The listing builds one solid part. Answer for the finished solid, in the listing's coordinates (mm). Coordinates: 2 decimals unless noted, no trailing zeros. Answer as a JSON object with one key per item and string values. Group by question number.
from build123d import *

# Parameters (mm, degrees)
BOSS_EXTRUDE1_DEPTH         = 3.175
F_1_4_0_25_DIAMETER_HOLE1_D = 6.35
FILLET1_R                   = 3.175


with BuildPart() as part:
    # Sketch1 → Boss-Extrude1 (new body)
    with BuildSketch(Plane(origin=(0, 0, 0), x_dir=(0, 0, -1), z_dir=(1, 0, 0))):
        Polygon((0, 0), (0, 1016), (524.232817332, 1016), (806.45, 733.782817332), (806.45, 0), align=None)
    extrude(amount=BOSS_EXTRUDE1_DEPTH)

    # 1/4 (0.25) Diameter Hole1 (through all)
    with Locations(Plane(origin=(3.175, 0, 0), x_dir=(0, 0, -1), z_dir=(1, 0, 0))):
        with Locations((95.25, 908.05), (68.2625, 152.4), (68.2625, 508), (68.2625, 863.6), (149.225, 947.7375), (415.925, 947.7375), (736.6, 155.575), (736.6, 612.775), (706.130949904, 735.319050096), (526.525827482, 914.924172518), (95.25, 266.7), (95.25, 311.15), (95.25, 863.6)):
            Hole(F_1_4_0_25_DIAMETER_HOLE1_D / 2)

    # Fillet1
    fillet1_edges = [part.edges().sort_by_distance(p)[0] for p in [
        (1.5875, 0, 0),
        (1.5875, 1016, 0),
        (1.5875, 1016, -524.232817332),
        (1.5875, 733.782817332, -806.45),
        (1.5875, 0, -806.45),
    ]]
    fillet(fillet1_edges, radius=FILLET1_R)


solid = part.part
Item 1: A cutting plane is placed at A-A, the plane x = 1.2. State how many separate pieces and enclosed holes the cut face has, and give its area (3 significant figures).
Item 2: Consider L1, parallel to Z at x = 1.35, y = 863.6 (1 decimal); L2, parallel to Z at x = 1.9, y = 311.15 (3 decimals); L3, parallel to Z at x = 0.35, y = 936.5. Determine where each line is inside the solid, lowest interval first. Write a range as from..to.
Item 3: Flat-ended cylindrical pins translate along their axes: pin 1 Ø4 at (y, z) = (947.74, -149.22) entering from -X; pin 2 Ø1 at (y, z) = (576.5, -409) entering from -X. Find the tip coordinate at first contact, or state that the pin passes through.
Answer:
{
 "1": {"separate pieces": "1", "enclosed holes": "13", "area": "779,000 mm2"},
 "2": {"L1": "-676.6..-98.4, -92.1..-71.4, -65.1..0", "L2": "-806.45..-98.425, -92.075..0", "L3": "-603.73..0"},
 "3": {"pin 1": "through", "pin 2": "x = 0"}
}
